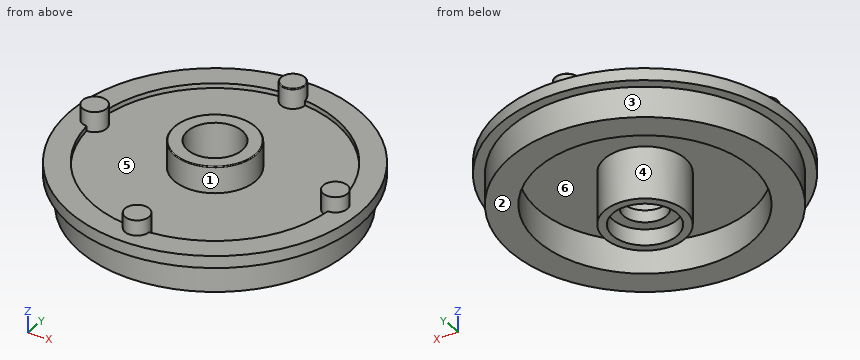
```python
from build123d import *

# Parameters (mm, degrees)
SKETCH1_R           = 16.75
BOSS_EXTRUDE1_DEPTH = 3.8
SKETCH2_R           = 18
BOSS_EXTRUDE2_DEPTH = 1.5
SKETCH3_R           = 13.25
CUT_EXTRUDE1_DEPTH  = 4
SKETCH4_R           = 5
BOSS_EXTRUDE3_DEPTH = 6.5
SKETCH5_R           = 4
CUT_EXTRUDE2_DEPTH  = 2
SKETCH7_R           = 15.1
CUT_EXTRUDE3_DEPTH  = 0.6
SKETCH8_R           = 5.05
BOSS_EXTRUDE4_DEPTH = 3.3
SKETCH6_R           = 2.65
CUT_EXTRUDE4_DEPTH  = 9.5
SKETCH9_R           = 3.4
CUT_EXTRUDE5_DEPTH  = 7
SKETCH10_R          = 1.5
BOSS_EXTRUDE5_DEPTH = 2.5
FILLET2_R           = 0.1
FILLET3_R           = 0.1
CIRPATTERN1_COUNT   = 4


with BuildPart() as part:
    # Sketch1 → Boss-Extrude1 (new body)
    with BuildSketch(Plane.XY):
        Circle(SKETCH1_R)
    extrude(amount=BOSS_EXTRUDE1_DEPTH)

    # Sketch2 → Boss-Extrude2 (add)
    with BuildSketch(Plane.XY.offset(3.8)):
        Circle(SKETCH2_R)
    extrude(amount=BOSS_EXTRUDE2_DEPTH)

    # Sketch3 → Cut-Extrude1 (cut)
    with BuildSketch(Plane(origin=(0, 0, 0), x_dir=(-1, 0, 0), z_dir=(0, 0, -1))):
        Circle(SKETCH3_R)
    extrude(amount=-CUT_EXTRUDE1_DEPTH, mode=Mode.SUBTRACT)

    # Sketch4 → Boss-Extrude3 (add)
    with BuildSketch(Plane(origin=(0, 0, 4), x_dir=(-1, 0, 0), z_dir=(0, 0, -1))):
        Circle(SKETCH4_R)
    extrude(amount=BOSS_EXTRUDE3_DEPTH)

    # Sketch5 → Cut-Extrude2 (cut)
    with BuildSketch(Plane(origin=(0, 0, -2.5), x_dir=(-1, 0, 0), z_dir=(0, 0, -1))):
        Circle(SKETCH5_R)
    extrude(amount=-CUT_EXTRUDE2_DEPTH, mode=Mode.SUBTRACT)

    # Sketch7 → Cut-Extrude3 (cut)
    with BuildSketch(Plane.XY.offset(5.3)):
        Circle(SKETCH7_R)
    extrude(amount=-CUT_EXTRUDE3_DEPTH, mode=Mode.SUBTRACT)

    # Sketch8 → Boss-Extrude4 (add)
    with BuildSketch(Plane.XY.offset(4.7)):
        Circle(SKETCH8_R)
    extrude(amount=BOSS_EXTRUDE4_DEPTH)

    # Sketch6 → Cut-Extrude4 (cut, through all)
    with BuildSketch(Plane(origin=(0, 0, -0.5), x_dir=(-1, 0, 0), z_dir=(0, 0, -1))):
        Circle(SKETCH6_R)
    extrude(amount=-CUT_EXTRUDE4_DEPTH, mode=Mode.SUBTRACT)

    # Sketch9 → Cut-Extrude5 (cut)
    with BuildSketch(Plane.XY.offset(8)):
        Circle(SKETCH9_R)
    extrude(amount=-CUT_EXTRUDE5_DEPTH, mode=Mode.SUBTRACT)

    # Sketch10 → Boss-Extrude5 (add)
    with BuildSketch(Plane.XY.offset(4.7)):
        with Locations((0, 15)):
            Circle(SKETCH10_R)
    boss_extrude5 = extrude(amount=BOSS_EXTRUDE5_DEPTH)

    # Fillet2
    fillet2_edges = [part.edges().sort_by_distance(p)[0] for p in [
        (-1.5, 15, 7.2),
    ]]
    fillet(fillet2_edges, radius=FILLET2_R)

    # Fillet3
    fillet3_edges = [part.edges().sort_by_distance(p)[0] for p in [
        (-5.05, 0, 8),
    ]]
    fillet(fillet3_edges, radius=FILLET3_R)

    # CirPattern1: Boss-Extrude5 ×4 about axis
    cirpattern1_axis = Axis((0, 0, 0), (0, 0, 1))
    for i in range(1, CIRPATTERN1_COUNT):
        add(boss_extrude5.rotate(cirpattern1_axis, i * 360 / CIRPATTERN1_COUNT))


solid = part.part
```
Model file for the job. Use its own axes, mm. Face numbers are marked on the shaded views. A direction names the side the tool comes from. Coordinates: 2 decimals unless noted, no trailing zeros. Order: outer loops, then holes, each group sorted by start corner. A loop starts at its lowest first (then second) coordinate and runs counter-clockwise, first axis right, second up. Notation, with made-up numbers: (58, -13.75) -> (110, -13.75) arc R5 cw to (110, -7.75) -> close; hole circle Ø9 at (57, 76.25). An arc over 180 degrees is marked (long way). Answer as a JSON object with one key per item and string values. Group by question number.
1) Cut at A-A, the plane z = 3. Write the cut outline in (x, y), then the cut area to 3 significant figures.
2) Flat gauge pins, fed straight in: pin 1 (2 mm diameter, centred on x = -1.5, y = 1, fed in from +Z); pin 2 (16 mm diameter, centred on x = 0, y = 0, fed in from +Z); pin 3 (2 mm diameter, centred on x = 5, z = 3, fed in from -Y); pin 4 (0.9 mm diameter, centred on x = 0, y = -15.5, fed in from +Z). Where does each tip first touch, or does it go through?
3) Which spindle directions (+Z, -Z, +X, -X, +Y, -Y) get a long thin tool onto all of the face, cutting with end or side? Do the marked faces 5 and 6. Say none if no direction does.
4) Cut at C-C, the plane x = 6.5. Write the cut outline in (y, z), then the cut area to 3 significant figures.
5) Cut at B-B, the plane y = 10. Write the cut outline in (x, z), then the cut area to 3 significant figures.
6) Pull direction X, two halves, no side cores. Call the marked faces 1, 2, 3 and 4: +X half, -X half, draft (parallel to the pull), parting line (faces both ways), or undercut.
7) Drill centre lines: L1, parallel to Y at x = 0, z = -1.1; L2, parallel to Y at x = 0, z = 5.5; L3, parallel to Z at x = 8.5, y = 11.5. Where is each one in solid material? Low to high.
8) Cut at D-D, the plane z = -1.25. Write the cut outline in (x, y).
Check values:
{
 "1": {"outline": "circle Ø33.5 at (0, 0); circle Ø10 at (0, 0); hole circle Ø26.5 at (0, 0); hole circle Ø6.8 at (0, 0)", "area": "372 mm²"},
 "2": {"pin 1": "stops at z = 1", "pin 2": "stops at z = 8", "pin 3": "stops at y = -17.45", "pin 4": "stops at z = 7.2"},
 "3": {"face 5": "+Z", "face 6": "-Z"},
 "4": {"outline": "(-16.79, 3.8) -> (-15.44, 3.8) -> (-15.44, 0) -> (-11.55, 0) -> (-11.55, 4) -> (11.55, 4) -> (11.55, 0) -> (15.44, 0) -> (15.44, 3.8) -> (16.79, 3.8) -> (16.79, 5.3) -> (13.63, 5.3) -> (13.63, 4.7) -> (-13.63, 4.7) -> (-13.63, 5.3) -> (-16.79, 5.3) -> close", "area": "59.0 mm²"},
 "5": {"outline": "(-14.97, 3.8) -> (-13.44, 3.8) -> (-13.44, 0) -> (-8.69, 0) -> (-8.69, 4) -> (8.69, 4) -> (8.69, 0) -> (13.44, 0) -> (13.44, 3.8) -> (14.97, 3.8) -> (14.97, 5.3) -> (11.31, 5.3) -> (11.31, 4.7) -> (-11.31, 4.7) -> (-11.31, 5.3) -> (-14.97, 5.3) -> close", "area": "63.9 mm²"},
 "6": {"face 1": "undercut", "face 2": "draft", "face 3": "parting line", "face 4": "undercut"},
 "7": {"L1": "y = -5 to -4, 4 to 5", "L2": "y = -16.5 to -13.5, -5.05 to -3.4, 3.4 to 5.05, 13.5 to 16.5", "L3": "z = 0 to 4.7"},
 "8": {"outline": "circle Ø10 at (0, 0); hole circle Ø8 at (0, 0)"}
}
